from build123d import *

# Parameters (mm, degrees)
BOSS_EXTRUDE1_DEPTH       = 16
F_8_36_TAPPED_HOLE1_D     = 3.4544
F_8_36_TAPPED_HOLE1_DEPTH = 25
F_8_36_TAPPED_HOLE1_TIP   = 1.037806461


with BuildPart() as part:
    # Sketch1 → Boss-Extrude1 (new body)
    with BuildSketch(Plane.XY):
        with BuildLine():
            Line((5.452946738, 0.717894057), (8, -18.628896236))
            Line((8, -18.628896236), (18, -18.628896236))
            Line((18, -18.628896236), (18, 16.371103764))
            Line((18, 16.371103764), (-18, 16.371103764))
            Line((-18, 16.371103764), (-18, -18.628896236))
            Line((-18, -18.628896236), (-8, -18.628896236))
            Line((-8, -18.628896236), (-5.452946738, 0.717894057))
            ThreePointArc((-5.452946738, 0.717894057), (0, 5.5), (5.452946738, 0.717894057))
        make_face()
    extrude(amount=BOSS_EXTRUDE1_DEPTH)

    # #8-36 Tapped Hole1
    with Locations(Plane(origin=(0, 16.371103764, 0), x_dir=(1, 0, 0), z_dir=(0, 1, 0))):
        with Locations((-13, -8), (13, -8)):
            Hole(F_8_36_TAPPED_HOLE1_D / 2, depth=F_8_36_TAPPED_HOLE1_DEPTH)
            with Locations((0, 0, -(F_8_36_TAPPED_HOLE1_DEPTH + F_8_36_TAPPED_HOLE1_TIP / 2))):  # 118° drill point
                Cone(0, F_8_36_TAPPED_HOLE1_D / 2, F_8_36_TAPPED_HOLE1_TIP, mode=Mode.SUBTRACT)


solid = part.part
Verification items for the finished model (mm, model axes). A direction names the side the tool comes from. Coordinates: 2 decimals unless noted, no trailing zeros. Order: outer loops, then holes, each group sorted by start corner. A loop starts at its lowest first (then second) coordinate and runs counter-clockwise, first axis right, second up. Notation, with made-up numbers: (61.5, 33.5) -> (95.5, 33.5) arc R14 ccw to (95.5, 38.5) -> close; hole circle Ø10 at (37.25, 75). An arc over 180 degrees is marked (long way). Use CSV: the item, a comma, the result in double quotes. Start each with the question number.
Q1. Section check A-A, the plane y = -5. Record the cut outline in (x, z), and give its area (3 significant figures).
Q2. Depth check by flat-ended pin: P1, Ø3, axis at x = -8, y = -13, coming from the -Z side; P2, Ø1.5, axis at x = -4, y = -1, coming from the -Z side. Enter the tip coordinate at first touch or a pass-through.
Q3. Section check B-B, the plane y = 10.5. Record the cut outline in (x, z), and give its area (3 significant figures).
Q4. Section check D-D, the plane x = -0.5. Record the cut outline in (y, z), and give its area (3 significant figures).
Q5. Thickness scan on line 1 along X through (y, z) = (6.25, 8); line 2 along Z through (x, y) = (-13, 3); line 3 along X through (y, z) = (-1.25, 8). Record the ranges inside material, lowest first.
Q6. Section check C-C, the plane z = 1. Record the cut outline in (x, y), and give its area (3 significant figures).
Q7. Tool access check on faces 4 (the flat face through (18, -1, 8)), 5 (the cylindrical face through (14.726, 3.696, 7.924)), 6 (the flat face through (6.71, -8.82, 7.89)). Record the directions out of +Z, -Z, +X, -X, +Y, -Y that give a thin tool (end or side, any length) a straight path to the whole face; none if there is none.
Q8. Draft check along Z on faces 1 (the conical face through (-12.714, -9.486, 7.91)), 2 (the flat face through (-6.744, -9.091, 7.888)), 3 (the flat face through (0, 7, 16)). Enter one of: +Z half, -Z half, draft (parallel to the pull), parting line (faces both ways), or undercut.
Returned:
1,outline,"(-18, 0) -> (-6.21, 0) -> (-6.21, 16) -> (-18, 16) -> close; (6.21, 0) -> (18, 0) -> (18, 16) -> (6.21, 16) -> close; hole circle Ø3.45 at (-13, 8); hole circle Ø3.45 at (13, 8)"
1,area,"359 mm^2"
2,P1,"stops at z = 0"
2,P2,"passes through"
3,outline,"(-18, 0) -> (18, 0) -> (18, 16) -> (-18, 16) -> close; hole circle Ø3.45 at (-13, 8); hole circle Ø3.45 at (13, 8)"
3,area,"557 mm^2"
4,outline,"(5.48, 0) -> (16.37, 0) -> (16.37, 16) -> (5.48, 16) -> close"
4,area,"174 mm^2"
5,line 1,"x = -18 to -14.73, -11.27 to 11.27, 14.73 to 18"
5,line 2,"z = 0 to 6.27, 9.73 to 16"
5,line 3,"x = -18 to -14.73, -11.27 to -5.71, 5.71 to 11.27, 14.73 to 18"
6,outline,"(-18, -18.63) -> (-8, -18.63) -> (-5.45, 0.72) arc R5.5 cw to (5.45, 0.72) -> (8, -18.63) -> (18, -18.63) -> (18, 16.37) -> (-18, 16.37) -> close"
6,area,"960 mm^2"
7,face 4,"+Z, -Z, +X, +Y, -Y"
7,face 5,"+Y"
7,face 6,"+Z, -Z, -Y"
8,face 1,"undercut"
8,face 2,"draft"
8,face 3,"+Z half"
